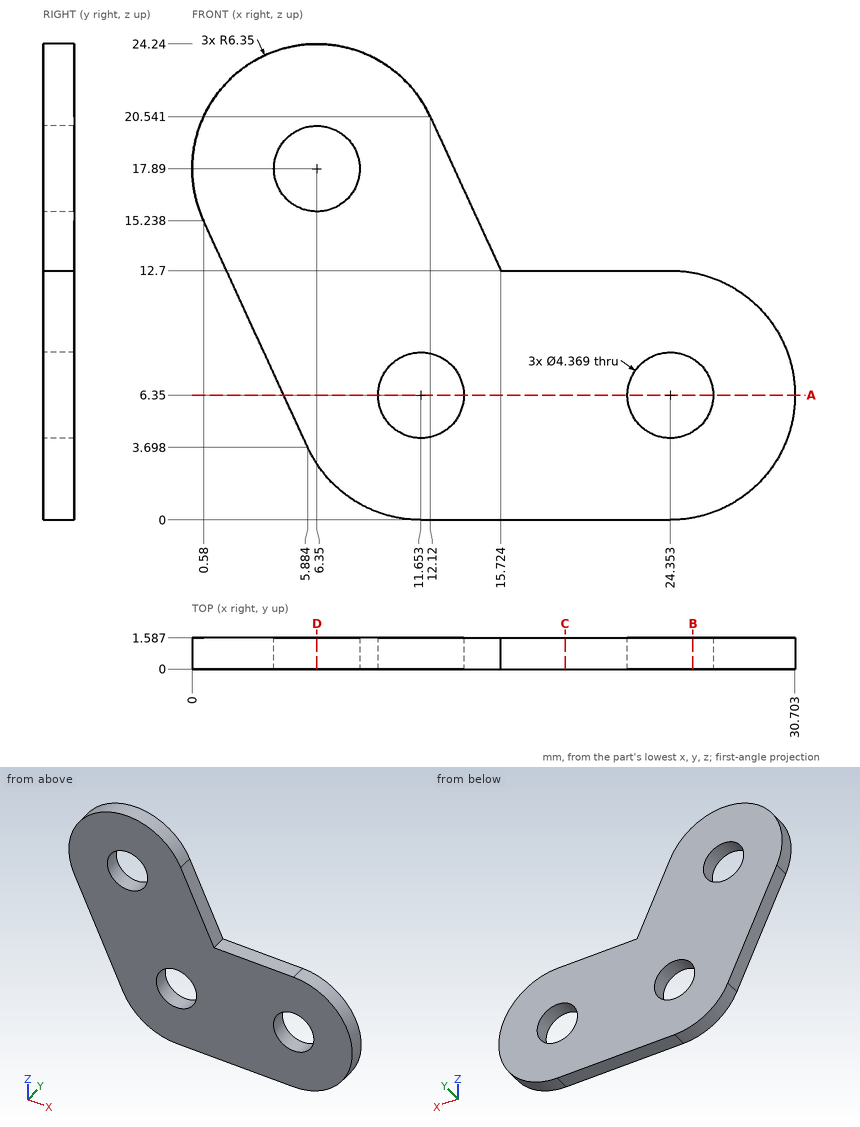
Study the drawing (mm; zero at the part's minimum x, y, z) and answer. Give positions to 0.01 mm unless a question says otherwise; leave off trailing zeros. Write each loop counter-clockwise with the first axis right and the second up, starting at its lowest first coordinate (ties: lowest second). Pieces come first, ordered by that corner, then holes. Notation, with made-up numbers: (35.25, 65.5) -> (47.25, 65.5) arc R21 cw to (47.25, 70.5) -> close; hole circle Ø2 at (-21, 1.25). An arc over 180 degrees is marked (long way). Write item = value, one per line. Start each with the question number.
1) Straight lines are drawn through the part: line 1 along X through (y, z) = (0.2, 6.25) (1 decimal); line 2 along X through (y, z) = (0.5, 5) (1 decimal); line 3 along Z through (x, y) = (22, 0.5). For each, find the intervals that lie inside material, in ascending order.
2) The part is cut by section B-B, the plane x = 25.5. Determine the outline of the cut face in (y, z) (1 decimal).
3) The part is cut by section D-D, the plane x = 6.35. Determine the outline of the cut face in (y, z) (1 decimal), and give its area (3 significant figures).
4) The part is cut by section C-C, the plane x = 19. Determine the outline of the cut face in (y, z).
5) The part is cut by section A-A, the plane z = 6.35. Determine the outline of the cut face in (x, y) (1 decimal).
Solutions:
q1.line_1 = 4.7 to 9.5, 13.8 to 22.2, 26.5 to 30.7
q1.line_2 = 5.3 to 9.9, 13.4 to 22.6, 26.1 to 30.6
q1.line_3 = 0 to 12.7
q2.outline = (0, 0.1) -> (1.6, 0.1) -> (1.6, 4.5) -> (0, 4.5) -> close; (0, 8.2) -> (1.6, 8.2) -> (1.6, 12.6) -> (0, 12.6) -> close
q3.outline = (0, 2.9) -> (1.6, 2.9) -> (1.6, 15.7) -> (0, 15.7) -> close; (0, 20.1) -> (1.6, 20.1) -> (1.6, 24.2) -> (0, 24.2) -> close
q3.area = 27.0 mm²
q4.outline = (0, 0) -> (1.59, 0) -> (1.59, 12.7) -> (0, 12.7) -> close
q5.outline = (4.7, 0) -> (9.5, 0) -> (9.5, 1.6) -> (4.7, 1.6) -> close; (13.8, 0) -> (22.2, 0) -> (22.2, 1.6) -> (13.8, 1.6) -> close; (26.5, 0) -> (30.7, 0) -> (30.7, 1.6) -> (26.5, 1.6) -> close
